Check sheet for the modelled part. Datum: model origin and axes. Units: mm. A direction names the side the tool comes from. Give positions to 0.01 mm unless a question says otherwise; leave off trailing zeros. Loops run counter-clockwise (first coordinate to the right, second up) from the corner with the lowest first, then second, coordinate; pieces in that order, holes last. Notation, with made-up numbers: (-18, 46.5) - (-14, 46.5) arc R14 ccw to (-14, 57.5) - close; hole circle Ø9 at (-14.75, 6.5). An arc over 180 degrees is marked (long way). Answer in a Markdown table with one row per item. Add a question column.
(1) Thickness scan on L1, parallel to X at y = -3.75, z = 2.25; L2, parallel to Y at x = -6.2, z = 4.55; L3, parallel to X at y = -2.5, z = 1. Record the ranges inside material, lowest first.
(2) Sectioned sample at C-C on z = 7. Enter the section's corners in (x, y).
(3) Draft check along Y on faces 1 (the face through (7.3, -3.8, 3)), 2 (the face through (-7, -7.5, 4)), 3 (the face through (11.37, -3.7, 8.22)). Enter one of: released by +Y, released by -Y, zero draft, split by the parting line, or undercut.
(4) Sectioned sample at D-D on y = -6. Enter the section's corners in (x, z), then the cut area to 3 significant figures.
(5) Sectioned sample at A-A on x = -6.2. Enter the section's corners in (y, z).
(6) Set-up check for faces 4 (the face through (-7, 0, 4)), 5 (the face through (-2.5, -3.7, 9.5)), 6 (the face through (-4, -4, 3.2)): record each of +Z, -Z, +X, -X, +Y, -Y from which the full face is reachable in a straight line by a thin tool's end or side.
(7) Sectioned sample at B-B on x = 5.5. Enter the section's corners in (y, z).
(8) Go/stop test with flat-tipped pins: P1, Ø4, axis at x = -6.2, y = -3.75, coming from the -Z side; P2, Ø2, axis at x = -6, z = 7.5, coming from the -Y side; P3, Ø1.5, axis at y = -1.5, z = 6.5, coming from the -X side; P4, Ø1.2, axis at y = -3, z = 6, coming from the -X side. Record where each tip stops, or that it passes through.
from build123d import *

# Parameters (mm, degrees)
F1_DEPTH     = 7.5
F2_R         = 1.6
F3_DEPTH     = 5.001
F4_R         = 2.75
F4_R_2       = 1.6
F5_DEPTH     = 3.2
F6_R         = 5
F7_SIZE      = 1
F8_DEPTH     = 12
F9_W         = 6.4
F9_H         = 5
F10_DEPTH    = 7.501
F11_SIZE     = 1
F12_T1_DEPTH = 28.5416254125
F13_R        = 1.6
F14_DEPTH    = 5.001
F15_R        = 2.75
F15_R_2      = 1.6
F16_DEPTH    = 3


# Not quite as in the source:
# - a fillet or chamfer that OpenCascade refuses, or shapes differently, is made with other operations: its cross-section is extruded or revolved along the edge and cut away or added


with BuildPart() as f1:
    # F0 (on Front) → F1 (new body)
    with BuildSketch(Plane.XZ):
        Polygon((-24.524355653, 0), (0, 0), (0, 10), (-3, 10), (-3, 5), (-9.4, 5), (-9.4, 10), (-12.4, 10), (-24.524355653, 3), align=None)
    extrude(amount=F1_DEPTH)

    # F2 (on face) → F3 (cut, through all)
    with BuildSketch(Plane.XY.offset(5)):
        with Locations((-6.2, -3.75)):
            Circle(F2_R)
    extrude(amount=-F3_DEPTH, mode=Mode.SUBTRACT)

    # F4 (on face) → F5 (cut)
    with BuildSketch(Plane(origin=(0, 0, 0), x_dir=(1, 0, 0), z_dir=(0, 0, -1))):
        with Locations((-6.2, 3.75)):
            Circle(F4_R)
        with Locations((-6.2, 3.75)):
            Circle(F4_R_2, mode=Mode.SUBTRACT)
    extrude(amount=-F5_DEPTH, mode=Mode.SUBTRACT)

    # F6
    f6_edges = [f1.edges().sort_by_distance(p)[0] for p in [
        (-12.4, -3.75, 10),
        (-24.524356, -3.75, 3),
    ]]
    fillet(f6_edges, radius=F6_R)

    # F7
    f7_edges = [f1.edges().sort_by_distance(p)[0] for p in [
        (-9.4, -3.75, 10),
        (-3, -3.75, 10),
    ]]
    chamfer(f7_edges, length=F7_SIZE)

    # F8 (add): a face of the model
    f8_faces = [f1.faces().sort_by_distance(p)[0] for p in [
        (0, -3.75, 5),
    ]]
    extrude(f8_faces, amount=F8_DEPTH)

    # F9 (on face) → F10 (cut, through all)
    with BuildSketch(Plane.XZ.offset(7.5)):
        with Locations((5.5, 7.5)):
            Rectangle(F9_W, F9_H)
    extrude(amount=-F10_DEPTH, mode=Mode.SUBTRACT)

    # F11
    f11_edges = [f1.edges().sort_by_distance(p)[0] for p in [
        (2.3, -3.75, 10),
        (8.7, -3.75, 10),
    ]]
    chamfer(f11_edges, length=F11_SIZE)

    # F12: fillet of radius 5 on 1 edges, made by hand

    # F12_s2 → F12_t1 (cut)
    with BuildSketch(Plane.XZ.offset(-10.5208127063)):
        with BuildLine():
            ThreePointArc((9.7, 10), (11.3874821937, 8.1895906792), (12, 5.7916749175))
            Line((12, 5.7916749175), (12, 10))
            Line((12, 10), (9.7, 10))
        make_face()
    extrude(amount=F12_T1_DEPTH, mode=Mode.SUBTRACT)

    # F13 (on face) → F14 (cut, through all)
    with BuildSketch(Plane.XY.offset(5)):
        with Locations((5.5, -3.75)):
            Circle(F13_R)
    extrude(amount=-F14_DEPTH, mode=Mode.SUBTRACT)

    # F15 (on face) → F16 (cut)
    with BuildSketch(Plane(origin=(0, 0, 0), x_dir=(1, 0, 0), z_dir=(0, 0, -1))):
        with Locations((5.5, 3.75)):
            Circle(F15_R)
        with Locations((5.5, 3.75)):
            Circle(F15_R_2, mode=Mode.SUBTRACT)
    extrude(amount=-F16_DEPTH, mode=Mode.SUBTRACT)


solid = f1.part
Reply:
| question | item | result |
|---|---|---|
| 1 | L1 | -24.04 to -8.95, -3.45 to 2.75, 8.25 to 12 |
| 1 | L2 | -7.5 to -5.35, -2.15 to 0 |
| 1 | L3 | -24.45 to -8.65, -3.75 to 3.05, 7.95 to 12 |
| 2 | outline | (-17.6, -7.5) - (-9.4, -7.5) - (-9.4, 0) - (-17.6, 0) - close; (-3, -7.5) - (2.3, -7.5) - (2.3, 0) - (-3, 0) - close; (8.7, -7.5) - (11.85, -7.5) - (11.85, 0) - (8.7, 0) - close |
| 3 | face 1 | undercut |
| 3 | face 2 | released by -Y |
| 3 | face 3 | zero draft |
| 4 | outline | (-24.52, 0) - (-7.78, 0) - (-7.78, 3.2) - (-4.62, 3.2) - (-4.62, 0) - (3.92, 0) - (3.92, 3) - (7.08, 3) - (7.08, 0) - (12, 0) - (12, 5.79) arc R5 ccw to (9.7, 10) - (8.7, 9) - (8.7, 5) - (2.3, 5) - (2.3, 9) - (1.3, 10) - (-2, 10) - (-3, 9) - (-3, 5) - (-9.4, 5) - (-9.4, 9) - (-10.4, 10) - (-11.06, 10) arc R5 ccw to (-13.56, 9.33) - (-22.02, 4.44) arc R5 ccw to (-24.52, 0.11) - close |
| 4 | area | 233 mm^2 |
| 5 | outline | (-7.5, 0) - (-6.5, 0) - (-6.5, 3.2) - (-5.35, 3.2) - (-5.35, 5) - (-7.5, 5) - close; (-2.15, 3.2) - (-1, 3.2) - (-1, 0) - (0, 0) - (0, 5) - (-2.15, 5) - close |
| 6 | face 4 | +Z, -Z, +X, -X, +Y |
| 6 | face 5 | +Z, +Y, -Y |
| 6 | face 6 | -Z |
| 7 | outline | (-7.5, 0) - (-6.5, 0) - (-6.5, 3) - (-5.35, 3) - (-5.35, 5) - (-7.5, 5) - close; (-2.15, 3) - (-1, 3) - (-1, 0) - (0, 0) - (0, 5) - (-2.15, 5) - close |
| 8 | P1 | z = 3.2 |
| 8 | P2 | through |
| 8 | P3 | x = -19.76 |
| 8 | P4 | x = -20.37 |
